from build123d import *

# Parameters (mm, degrees)
BOSS_EXTRUDE1_DEPTH                               = 5
BOSS_EXTRUDE2_DEPTH                               = 4.4
CUT_EXTRUDE2_START                                = -5
SKETCH4_R                                         = 4.9
CUT_EXTRUDE2_DEPTH                                = 1.5
CSK_FOR_8_FLAT_HEAD_SOCKET_CAP_SCREW1_D           = 4.9149
CSK_FOR_8_FLAT_HEAD_SOCKET_CAP_SCREW1_DEPTH       = 68.34
CSK_FOR_8_FLAT_HEAD_SOCKET_CAP_SCREW1_CSINK_D     = 9.1186
CSK_FOR_8_FLAT_HEAD_SOCKET_CAP_SCREW1_CSINK_ANGLE = 82
CSK_FOR_8_FLAT_HEAD_SOCKET_CAP_SCREW1_TIP         = 1.476584928


with BuildPart() as part:
    # Sketch1 → Boss-Extrude1 (new body)
    with BuildSketch(Plane(origin=(0, 0, 0), x_dir=(1, 0, 0), z_dir=(0, 1, 0))):
        with BuildLine():
            Line((-60, -30), (-60, 40))
            ThreePointArc((-60, 40), (-54.142135624, 54.142135624), (-40, 60))
            Line((-40, 60), (40, 60))
            ThreePointArc((40, 60), (54.142135624, 54.142135624), (60, 40))
            Line((60, 40), (60, -30))
            ThreePointArc((60, -30), (54.142135624, -44.142135624), (40, -50))
            Line((40, -50), (-40, -50))
            ThreePointArc((-40, -50), (-54.142135624, -44.142135624), (-60, -30))
        make_face()
    extrude(amount=BOSS_EXTRUDE1_DEPTH)

    # Sketch1<5> → Boss-Extrude2 (add)
    with BuildSketch(Plane(origin=(0, 0, 0), x_dir=(1, 0, 0), z_dir=(0, 1, 0))):
        with BuildLine():
            Line((-39.4, -22.6), (41.9, -22.6))
            Line((41.9, -22.6), (41.9, -32))
            ThreePointArc((41.9, -32), (39.146803743, -38.646803743), (32.5, -41.4))
            Line((32.5, -41.4), (-30, -41.4))
            ThreePointArc((-30, -41.4), (-36.646803743, -38.646803743), (-39.4, -32))
            Line((-39.4, -32), (-39.4, -22.6))
        make_face()
        with BuildLine():
            Line((3.1, 54.4), (3.1, 30.6))
            Line((3.1, 30.6), (41.9, 30.6))
            Line((41.9, 30.6), (41.9, 43))
            ThreePointArc((41.9, 43), (38.561017306, 51.061017306), (30.5, 54.4))
            Line((30.5, 54.4), (3.1, 54.4))
        make_face()
    extrude(amount=-BOSS_EXTRUDE2_DEPTH)

    # Sketch4 → Cut-Extrude2 (cut)
    with BuildSketch(Plane(origin=(0, 5, 0), x_dir=(1, 0, 0), z_dir=(0, 1, 0)).offset(CUT_EXTRUDE2_START)):
        with Locations((-20.2, -7)):
            Circle(SKETCH4_R)
        with Locations((-43.84, -2.83)):
            Circle(SKETCH4_R)
        with Locations((3.44, 12.83)):
            Circle(SKETCH4_R)
        with Locations((44.41, -4.14)):
            Circle(SKETCH4_R)
        with Locations((27.44, 12.83)):
            Circle(SKETCH4_R)
    extrude(amount=CUT_EXTRUDE2_DEPTH, mode=Mode.SUBTRACT)

    # CSK for #8 Flat Head Socket Cap Screw1
    with Locations(Plane(origin=(50, 5, 40), x_dir=(0, 0, 1), z_dir=(0, 1, 0))):
        with Locations((0, 0), (-90, 0), (-90, -100), (0, -100)):
            CounterSinkHole(CSK_FOR_8_FLAT_HEAD_SOCKET_CAP_SCREW1_D / 2, CSK_FOR_8_FLAT_HEAD_SOCKET_CAP_SCREW1_CSINK_D / 2, depth=CSK_FOR_8_FLAT_HEAD_SOCKET_CAP_SCREW1_DEPTH, counter_sink_angle=CSK_FOR_8_FLAT_HEAD_SOCKET_CAP_SCREW1_CSINK_ANGLE)
            with Locations((0, 0, -(CSK_FOR_8_FLAT_HEAD_SOCKET_CAP_SCREW1_DEPTH + CSK_FOR_8_FLAT_HEAD_SOCKET_CAP_SCREW1_TIP / 2))):  # 118° drill point
                Cone(0, CSK_FOR_8_FLAT_HEAD_SOCKET_CAP_SCREW1_D / 2, CSK_FOR_8_FLAT_HEAD_SOCKET_CAP_SCREW1_TIP, mode=Mode.SUBTRACT)


solid = part.part
Could you check a few things on this model? Use its own coordinates, in mm. A direction names the side the tool comes from. Round coordinates to 2 decimals unless told otherwise and drop trailing zeros. Write each loop counter-clockwise with the first axis right and the second up, starting at its lowest first coordinate (ties: lowest second). Pieces come first, ordered by that corner, then holes. Notation, with made-up numbers: (15, -31.75) - (24, -31.75) arc R31 cw to (24, 1.25) - close; hole circle Ø10 at (-1.75, -38). An arc over 180 degrees is marked (long way). Put each result on its own line as item: value. Start each with the question number.
(1) I want a section at D-D, the plane z = 40. Please give me the cut outline in (x, y).
(2) Thinking about a two-plate mould opening in Z: for faces 1 (the flat face through (22, -2, -30.6)), 2 (the cylindrical face through (38.65, -2.17, -50.97)), 3 (the flat face through (41.9, -2, 27)), 4 (the cylindrical face through (-53.986, 2.465, 44.297)), which applies, released by +Z, released by -Z, zero draft, split by the parting line, or undercut?
(3) I want a section at B-B, the plane y = -2.5. Please give me the cut outline in (x, z).
(4) I want a section at A-A, the plane x = 11.5. Please give me the cut outline in (y, z), plus the area to 3 significant figures.
(5) For faces 5 (the flat face through (3.1, -2, -43)), 6 (the cylindrical face through (-36.57, -2.17, 38.72)), 7 (the flat face through (44, 1.5, 4)), which set-ups out of +Z, -Z, +X, -X, +Y, -Y let a thin tool reach every point of the face, with its end or its side?
(6) Will these pins go through, and if not, where does the flat tip stop? pin 1 (1 mm diameter, centred on x = 33.5, y = -2.5, fed in from +Z); pin 2 (3 mm diameter, centred on x = 50, z = -50, fed in from -Y); pin 3 (2 mm diameter, centred on x = 2.5, y = -2.5, fed in from -Z); pin 4 (3.5 mm diameter, centred on y = -3.5, z = 25, fed in from -X).
(7) I want a section at C-C, the plane z = 24. Please give me the cut outline in (x, y).
(8) I need wall thicknesses on probe 1 along X at (y, z) = (0.8, 7); probe 2 along X at (y, z) = (0.4, 2.83); probe 3 along Y at (x, z) = (-48, -44.5). Which ranges of each line are inside material? Lowest first, please.
Here are the results:
1. outline: (-57.32, 0) - (-52.46, 0) - (-52.46, 2.58) - (-54.56, 5) - (-57.32, 5) - close; (-47.54, 0) - (-34.94, 0) - (-34.94, -4.4) - (37.44, -4.4) - (37.44, 0) - (47.54, 0) - (47.54, 2.58) - (45.44, 5) - (-45.44, 5) - (-47.54, 2.58) - close; (52.46, 0) - (57.32, 0) - (57.32, 5) - (54.56, 5) - (52.46, 2.58) - close
2. face 1: undercut
2. face 2: released by -Z
2. face 3: zero draft
2. face 4: released by +Z
3. outline: (-39.4, 22.6) - (41.9, 22.6) - (41.9, 32) arc R9.4 ccw to (32.5, 41.4) - (-30, 41.4) arc R9.4 ccw to (-39.4, 32) - close; (3.1, -54.4) - (30.5, -54.4) arc R11.4 ccw to (41.9, -43) - (41.9, -30.6) - (3.1, -30.6) - close
4. outline: (-4.4, -54.4) - (0, -54.4) - (0, -60) - (5, -60) - (5, 50) - (0, 50) - (0, 41.4) - (-4.4, 41.4) - (-4.4, 22.6) - (0, 22.6) - (0, -30.6) - (-4.4, -30.6) - close
4. area: 737 mm^2
5. face 5: -Z, -X, -Y
5. face 6: +Z, -X, -Y
5. face 7: -Y
6. pin 1: stops at z = 41.39
6. pin 2: passes through
6. pin 3: stops at z = -54.4
6. pin 4: stops at x = -39.4
7. outline: (-60, 0) - (-39.4, 0) - (-39.4, -4.4) - (41.9, -4.4) - (41.9, 0) - (60, 0) - (60, 5) - (-60, 5) - close
8. probe 1: x = -60 to -46.41, -41.27 to -25.1, -15.3 to 40.43, 48.39 to 60
8. probe 2: x = -60 to -48.74, -38.94 to -22.77, -17.63 to 39.69, 49.13 to 60
8. probe 3: y = 0 to 5
